Geometry check sheet. Reference: the model listing, model coordinates, mm. A direction names the side the tool comes from. Round coordinates to 2 decimals unless told otherwise and drop trailing zeros. Loops run counter-clockwise (first coordinate to the right, second up) from the corner with the lowest first, then second, coordinate; pieces in that order, holes last. Notation, with made-up numbers: M 5.25,0 L 51.25,0 A21 cw 51.25,32 Z; hole C -34.75,-18.75 d5. An arc over 180 degrees is marked long. Use one line per item in the form item = value. Start each with the question number.
1. Material ranges on line 1 (Y direction, x = 12.5, z = -11.6); line 2 (Y direction, x = -9.25, z = 0.5); line 3 (Y direction, x = -0.75, z = -4.25), recorded low to high.
2. Cross-section at B-B (y = 4.85). Record the boundary of the cut face in (x, z).
3. Cross-section at C-C (y = 13). Record the boundary of the cut face in (x, z).
4. Draft check along Z on faces 1 (the flat face through (8, 2, 7)), 2 (the cylindrical face through (8.112, 9.415, 12.699)), 3 (the flat face through (8, 5, -13)). Enter one of: pulls with the +Z half, pulls with the -Z half, needs draft (parallel to the pull), parting line crosses it, or undercut.
5. Set-up check for faces 4 (the flat face through (1, 17, 0.7)), 5 (the cylindrical face through (-7, 2, 0)), 6 (the cylindrical face through (0.865, 15.876, 2.747)), 7 (the flat face through (8, 5, 10)): record each of +Z, -Z, +X, -X, +Y, -Y from which the full face is reachable in a straight line by a thin tool's end or side.
6. Cross-section at A-A (x = 12.5). Record the boundary of the cut face in (y, z), then the cut area to 3 significant figures.
7. Go/stop test with flat-tipped pins: pin 1 (4.5 mm diameter, centred on x = 12.5, y = 4.85, fed in from -Z); pin 2 (4 mm diameter, centred on x = 11, z = 2, fed in from -Y); pin 3 (12 mm diameter, centred on y = 19.5, z = -7, fed in from -X); pin 4 (8 mm diameter, centred on y = 14.5, z = -3, fed in from +X). Record where each tip stops, or that it passes through.
```python
from build123d import *

# Parameters (mm, degrees)
BOSS_EXTRUDE1_DEPTH   = 3
BOSS_EXTRUDE2_DEPTH   = 3.7
BOSS_EXTRUDE3_DEPTH   = 3
SKETCH4_R             = 2.88
BOSS_EXTRUDE4_DEPTH   = 12
F_2_5MM_DOWEL_HOLE1_D = 2.5
SKETCH8_R             = 1.35
CUT_EXTRUDE1_DEPTH    = 38.455173265
FILLET1_R             = 1
FILLET2_R             = 1
CUT_EXTRUDE2_START    = -8
CUT_EXTRUDE2_DEPTH    = 8
FILLET3_R             = 0.5


with BuildPart() as part:
    # Sketch1 → Boss-Extrude1 (new body)
    with BuildSketch(Plane(origin=(0, 0, 0), x_dir=(1, 0, 0), z_dir=(0, 1, 0))):
        with BuildLine():
            Line((0, 13), (16, 13))
            Line((16, 13), (16, 7))
            Line((16, 7), (0, 7))
            ThreePointArc((0, 7), (-7, 0), (0, -7))
            Line((0, -7), (16, -7))
            Line((16, -7), (16, -13))
            Line((16, -13), (0, -13))
            ThreePointArc((0, -13), (-13, 0), (0, 13))
        make_face()
    extrude(amount=BOSS_EXTRUDE1_DEPTH)

    # Sketch2 → Boss-Extrude2 (add)
    with BuildSketch(Plane(origin=(0, 3, 0), x_dir=(1, 0, 0), z_dir=(0, 1, 0))):
        with BuildLine():
            Line((0, 13), (16, 13))
            Line((16, 13), (16, 10))
            Line((16, 10), (0, 10))
            ThreePointArc((0, 10), (-10, 0), (0, -10))
            Line((0, -10), (16, -10))
            Line((16, -10), (16, -13))
            Line((16, -13), (0, -13))
            ThreePointArc((0, -13), (-13, 0), (0, 13))
        make_face()
    extrude(amount=BOSS_EXTRUDE2_DEPTH)

    # Sketch3 → Boss-Extrude3 (add)
    with BuildSketch(Plane(origin=(0, 6.7, 0), x_dir=(1, 0, 0), z_dir=(0, 1, 0))):
        with BuildLine():
            Line((16, 13), (0, 13))
            ThreePointArc((0, 13), (-13, 0), (0, -13))
            Line((0, -13), (16, -13))
            Line((16, -13), (16, -7))
            Line((16, -7), (16, 7))
            Line((16, 7), (16, 13))
        make_face()
    extrude(amount=BOSS_EXTRUDE3_DEPTH)

    # Sketch4 → Boss-Extrude4 (add)
    with BuildSketch(Plane(origin=(0, 9.7, 0), x_dir=(1, 0, 0), z_dir=(0, 1, 0))):
        with Locations(Location((0, 0, 0), (0, 0, 270))):
            Circle(SKETCH4_R)
    extrude(amount=BOSS_EXTRUDE4_DEPTH)

    # Ø2.5mm Dowel Hole1 (through all)
    with Locations(Plane(origin=(-0.002429038, 18.104937254, 2.879998976), x_dir=(0.999999644325, 0, 0.000843415861), z_dir=(-0.000843415861, 0, 0.999999644325))):
        with Locations((0, 0)):
            Hole(F_2_5MM_DOWEL_HOLE1_D / 2)

    # Sketch8 → Cut-Extrude1 (cut, through all)
    with BuildSketch(Plane.XY.offset(13)):
        with Locations((12.5, 4.85)):
            Circle(SKETCH8_R)
    extrude(amount=-CUT_EXTRUDE1_DEPTH, mode=Mode.SUBTRACT)

    # Fillet1
    fillet1_edges = [part.edges().sort_by_distance(p)[0] for p in [
        (8, 0, -13),
        (8, 0, -7),
        (-7, 0, 0),
        (16, 4.85, 13),
        (-13, 9.7, 0),
        (8, 9.7, 13),
        (8, 9.7, -13),
        (8, 0, 7),
        (8, 0, 13),
        (-13, 0, 0),
    ]]
    fillet(fillet1_edges, radius=FILLET1_R)

    # Fillet2
    fillet2_edges = [part.edges().sort_by_distance(p)[0] for p in [
        (0, 9.7, -2.88),
    ]]
    fillet(fillet2_edges, radius=FILLET2_R)

    # Sketch10 → Cut-Extrude2 (cut)
    with BuildSketch(Plane(origin=(0, 21.7, 0), x_dir=(1, 0, 0), z_dir=(0, 1, 0)).offset(CUT_EXTRUDE2_START)):
        with BuildLine():
            Line((-2.793635624, 0.7), (2.793635624, 0.7))
            ThreePointArc((2.793635624, 0.7), (2.88, 0), (2.793635624, -0.7))
            Line((2.793635624, -0.7), (-2.793635624, -0.7))
            ThreePointArc((-2.793635624, -0.7), (-2.88, 0), (-2.793635624, 0.7))
        make_face()
    extrude(amount=CUT_EXTRUDE2_DEPTH, mode=Mode.SUBTRACT)

    # Fillet3
    fillet3_edges = [part.edges().sort_by_distance(p)[0] for p in [
        (0, 21.7, -2.88),
        (1.771778767, 21.7, 2.270506551),
    ]]
    fillet(fillet3_edges, radius=FILLET3_R)


solid = part.part
```
Reported:
q1.line_1 = 0 to 3.5, 6.2 to 9.7
q1.line_2 = 0 to 3, 6.7 to 9.7
q1.line_3 = 6.7 to 9.7
q2.outline = M 0,-13 L 11.15,-13 L 11.15,-10 L 0,-10 A10 cw 0,10 L 11.15,10 L 11.15,13 L 0,13 A13 ccw Z; M 13.85,-13 L 16,-13 L 16,-10 L 13.85,-10 Z; M 13.85,10 L 16,10 L 16,12 A1 ccw 15,13 L 13.85,13 Z
q3.outline = C 0,0 d5.76
q4.face_1 = undercut
q4.face_2 = pulls with the +Z half
q4.face_3 = pulls with the -Z half
q5.face_4 = +X, -X, +Y
q5.face_5 = +X, -Y
q5.face_6 = +Y
q5.face_7 = +X
q6.outline = M 0,-12 A1 ccw 1,-13 L 3.5,-13 L 3.5,-10 L 3,-10 L 3,-7 L 1,-7 A1 ccw 0,-8 Z; M 0,8 A1 ccw 1,7 L 3,7 L 3,10 L 3.5,10 L 3.5,13 L 1,13 A1 ccw 0,12 Z; M 6.2,-13 L 8.7,-13 A1 ccw 9.7,-12 L 9.7,12 A1 ccw 8.7,13 L 6.2,13 L 6.2,10 L 6.7,10 L 6.7,-10 L 6.2,-10 Z
q6.area = 119 mm²
q7.pin_1 = -13
q7.pin_2 = 6.7
q7.pin_3 = -2.7
q7.pin_4 = 2.88
